Autodesk Inventor part; units mm, degrees
ref_plane "Work Plane2" through (8.89, 0, 0) normal (1, 0, 0) x (0, 0, -1)
ref_plane "Work Plane1" through (-12.7, 0, 0) normal (1, 0, 0) x (0, 0, -1)
ref_plane "YZ Plane" through (0, 0, 0) normal (1, 0, 0) x (0, 1, 0)
sketch "Sketch1" plane through (0, 0, 0) normal (1, 0, 0) x (0, 1, 0)
  circle A0 centre (0, 0) radius 19.05
  dimension "d0" = 38.1
extrude "Extrusion1" add sketch "Sketch1" along normal blind 12.7
sketch "Sketch10" plane through (12.7, 0, 0) normal (1, 0, 0) x (0, 0, -1)
  point P0 (0, 0)
  point P1 (0, 0)
hole "Hole4" at (12.7, 0, 0) direction (-1, 0, 0) diameter 12.7 depth 3.81
ref_plane "Work Plane2" through (8.89, 0, 0) normal (1, 0, 0) x (0, 0, -1)
hole "Hole1" at (8.89, 0, 0) direction (-1, 0, 0) diameter 9.9219 depth 4.7625
ref_plane "Work Plane1" through (-12.7, 0, 0) normal (1, 0, 0) x (0, 0, -1)
sketch "Sketch5" plane through (0, 0, 0) normal (1, 0, 0) x (0, 1, 0)
  line L0 (0, 9) -> (0, -9)
  circle A0 centre (0, 0) radius 19.05
  line L1 (-10.795, 0) -> (10.795, 0)
  line L2 (-10.795, 8.89) -> (-10.795, -8.89)
  dimension "d37" = 18
  dimension "d45" = 21.59
  dimension "d46" = 17.78
hole "Hole2" at (0, 0, -9) direction (1, 0, 0) diameter 2.159 depth 8.8646 tip angle 118
sketch "Sketch6" plane through (0, 0, 0) normal (-1, 0, 0) x (0, 0, 1)
  circle A0 centre (0, 0) radius 0.5715
  dimension "d34" = 1.143
hole "Hole5" at (0, 0, 0) direction (1, 0, 0) diameter 1 end through all
mirror "Mirror1" about plane through (0, 0, 0) normal (0, 0, 1) of "Hole2"
hole "Hole3" at (0, -10.795, 8.89) at (0, -10.795, -8.89) direction (1, 0, 0) diameter 2.9464 end through all
mirror "Mirror2" about plane through (0, 0, 0) normal (0, 1, 0) of "Hole3"
sketch "Sketch9" plane through (0, 0, 0) normal (0, 1, 0) x (-1, 0, 0)
  line L0 (-11.4554, -7.9375) -> (-12.7, -7.9375)
  line L1 (-12.7, -7.9375) -> (-12.7, -10.4775)
  line L2 (-12.7, -10.4775) -> (-11.4554, -10.4775)
  line L3 (-11.4554, -10.4775) -> (-11.4554, -7.9375)
  line L4 (2.54, 0) -> (-15.24, 0)
  line L5 (-12.7, 19.05) -> (-12.7, -19.05)
  point P0 (0, 0)
  dimension "d55" = 2.54
  dimension "d56" = 1.2446
  dimension "d59" = 7.9375
revolve "Revolution1" cut sketch "Sketch9" angle 360 about axis through (-10, 0, 0) along (1, 0, 0)
properties part number "0.375 in hole" material "Aluminum 6061"
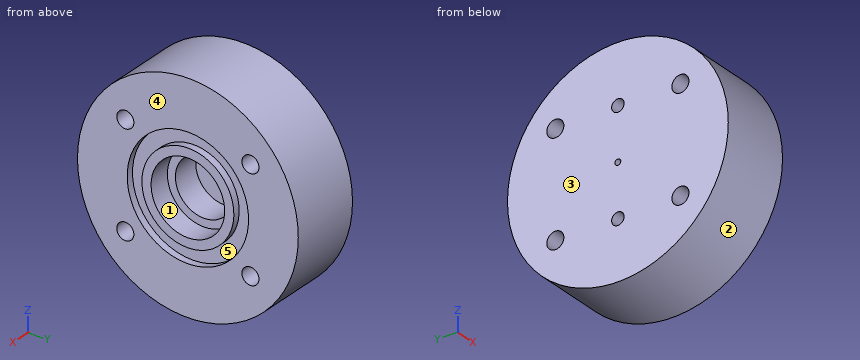
Part model, mm, in its own coordinate system. Face numbers are marked on the shaded views. A direction names the side the tool comes from. Coordinates: 2 decimals unless noted, no trailing zeros. Loops run counter-clockwise (first coordinate to the right, second up) from the corner with the lowest first, then second, coordinate; pieces in that order, holes last. Notation, with made-up numbers: (12.25, -35) -> (36.25, -35) arc R16 ccw to (36.25, -5) -> close; hole circle Ø7 at (31, -10.75). An arc over 180 degrees is marked (long way). Use a Markdown table: item, result. Add a question column.
Item 1: Band-saw the part on A-A on z = 0. Write the cut outline in (x, y), plus the area to 3 significant figures.
Item 2: Band-saw the part on B-B on x = 3.5. Give the number of separate pieces and of enclosed holes in the cut face, plus the area to 3 significant figures.
Item 3: Band-saw the part on D-D on z = -4. Write the cut outline in (x, y).
Item 4: Probe probe 1 along Z at (x, y) = (4.75, -10.5); probe 2 along Z at (x, y) = (7.2, 0); probe 3 along Z at (x, y) = (9.25, 11.5). List the from-to ranges inside material, lowest first.
Item 5: Pull direction Y, two halves, no side cores. Call the marked faces 1, 2 and 3: +Y half, -Y half, draft (parallel to the pull), parting line (faces both ways), or undercut.
Item 6: Band-saw the part on C-C on y = 2. Write the cut outline in (x, z), plus the area to 3 significant figures.
Item 7: Which spindle directions (+Z, -Z, +X, -X, +Y, -Y) get a long thin tool onto all of the face, cutting with end or side? Do the marked faces 4 and 5. Say none if no direction does.
Item 8: Flat gauge pins, fed straight in: P1, Ø6.5, axis at y = -4, z = -0.5, coming from the +X side; P2, Ø1.5, axis at x = 10, y = 15, coming from the +Z side; P3, Ø6, axis at y = 0, z = 0, coming from the +X side; P4, Ø1.7, axis at y = 0, z = -9, coming from the +X side. Where does each tip first touch, or does it go through?
Geometry says:
| question | item | result |
|---|---|---|
| 1 | outline | (0, -19.05) -> (12.7, -19.05) -> (12.7, -10.48) -> (11.46, -10.48) -> (11.46, -7.94) -> (12.7, -7.94) -> (12.7, -6.35) -> (8.89, -6.35) -> (8.89, -4.96) -> (4.13, -4.96) -> (4.13, -0.5) -> (0, -0.5) -> close; (0, 0.5) -> (4.13, 0.5) -> (4.13, 4.96) -> (8.89, 4.96) -> (8.89, 6.35) -> (12.7, 6.35) -> (12.7, 7.94) -> (11.46, 7.94) -> (11.46, 10.48) -> (12.7, 10.48) -> (12.7, 19.05) -> (0, 19.05) -> close |
| 1 | area | 378 mm² |
| 2 | separate pieces | 1 |
| 2 | enclosed holes | 7 |
| 2 | area | 1,100 mm² |
| 3 | outline | (0, -18.63) -> (12.7, -18.63) -> (12.7, -9.68) -> (11.46, -9.68) -> (11.46, -6.86) -> (12.7, -6.86) -> (12.7, -4.93) -> (8.89, -4.93) -> (8.89, -2.93) -> (4.13, -2.93) -> (4.13, 2.93) -> (8.89, 2.93) -> (8.89, 4.93) -> (12.7, 4.93) -> (12.7, 6.86) -> (11.46, 6.86) -> (11.46, 9.68) -> (12.7, 9.68) -> (12.7, 18.63) -> (0, 18.63) -> close |
| 4 | probe 1 | -15.9 to -10.33, -7.45 to 7.45, 10.33 to 15.9 |
| 4 | probe 2 | -19.05 to -10.08, -7.92 to -4.96, 4.96 to 7.92, 10.08 to 19.05 |
| 4 | probe 3 | -15.19 to -10.18, -7.6 to 7.6, 10.18 to 15.19 |
| 5 | face 1 | undercut |
| 5 | face 2 | parting line |
| 5 | face 3 | draft |
| 6 | outline | (0, -18.94) -> (12.7, -18.94) -> (12.7, -10.28) -> (11.46, -10.28) -> (11.46, -7.68) -> (12.7, -7.68) -> (12.7, -6.03) -> (8.89, -6.03) -> (8.89, -4.54) -> (4.13, -4.54) -> (4.13, 4.54) -> (8.89, 4.54) -> (8.89, 6.03) -> (12.7, 6.03) -> (12.7, 7.68) -> (11.46, 7.68) -> (11.46, 10.28) -> (12.7, 10.28) -> (12.7, 18.94) -> (0, 18.94) -> close |
| 6 | area | 386 mm² |
| 7 | face 4 | +Z, -Z, +X, +Y, -Y |
| 7 | face 5 | +X |
| 8 | P1 | x = 12.7 |
| 8 | P2 | z = 12.64 |
| 8 | P3 | x = 4.13 |
| 8 | P4 | x = 11.46 |
